Geometry check sheet. Reference: the model listing, model coordinates, mm. Round coordinates to 2 decimals unless told otherwise and drop trailing zeros. Order: outer loops, then holes, each group sorted by start corner. A loop starts at its lowest first (then second) coordinate and runs counter-clockwise, first axis right, second up. Notation, with made-up numbers: (-14.5, 46) - (9.5, 46) arc R21 ccw to (9.5, 73) - close; hole circle Ø9 at (56, 89). An arc over 180 degrees is marked (long way). Write each question's results on one line, items separated by ' | '.
```python
from build123d import *

# Parameters (mm, degrees)
SZKIC1_R                        = 3
DODANIE_WYCI_GNI_CIE1_DEPTH     = 65
DODANIE_WYCI_GNI_CIE2_START     = 65
SZKIC1_2_R                      = 3
DODANIE_WYCI_GNI_CIE2_DEPTH     = 120
SFAZOWANIE1_SIZE                = 1
SZKIC2_R                        = 1.05
WYTNIJ_WYCI_GNI_CIE1_DEPTH      = 4
WYTNIJ_WYCI_GNI_CIE1_DEPTH_BACK = 4


with BuildPart() as part:
    # Szkic1 → Dodanie-wyci_gni_cie1 (new body)
    with BuildSketch(Plane.XY):
        Circle(SZKIC1_R)
    extrude(amount=DODANIE_WYCI_GNI_CIE1_DEPTH)

    # Szkic1_2 → Dodanie-wyci_gni_cie2 (add)
    with BuildSketch(Plane.XY.offset(DODANIE_WYCI_GNI_CIE2_START)):
        Circle(SZKIC1_2_R)
    extrude(amount=-DODANIE_WYCI_GNI_CIE2_DEPTH)

    # Sfazowanie1
    sfazowanie1_edges = [part.edges().sort_by_distance(p)[0] for p in [
        (-3, 0, 65),
        (-3, 0, -55),
    ]]
    chamfer(sfazowanie1_edges, length=SFAZOWANIE1_SIZE)

    # Szkic2 → Wytnij-wyci_gni_cie1 (cut, two sides)
    with BuildSketch(Plane(origin=(0, 0, 0), x_dir=(1, 0, 0), z_dir=(0, 1, 0))) as wytnij_wyci_gni_cie1_sk:
        Circle(SZKIC2_R)
    extrude(amount=WYTNIJ_WYCI_GNI_CIE1_DEPTH, mode=Mode.SUBTRACT)
    extrude(wytnij_wyci_gni_cie1_sk.sketch, amount=-WYTNIJ_WYCI_GNI_CIE1_DEPTH_BACK, mode=Mode.SUBTRACT)


solid = part.part
```
(1) Section check B-B (z = 0). Record the cut outline in (x, y).
Answers follow:
outline: (-1.05, -2.81) - (-1.05, 2.81) arc R3 ccw to start; (1.05, -2.81) arc R3 ccw to (1.05, 2.81) - close
(2) Material ranges on line 1 (Z direction, x = 0, y = -1); line 2 (X direction, y = -2.25, z = 8.5); line 3 (X direction, y = -2.35, z = 0), recorded low to high.
Answers follow:
line 1: -55 to -1.05, 1.05 to 65 | line 2: -1.98 to 1.98 | line 3: -1.86 to -1.05, 1.05 to 1.86
(3) Section check C-C (z = 44). Record the cut outline in (x, y).
Answers follow:
outline: circle Ø6 at (0, 0)
(4) Section check A-A (x = 0). Record the cut outline in (y, z), then the cut area to 3 significant figures.
Answers follow:
outline: (-3, -54) - (-2, -55) - (2, -55) - (3, -54) - (3, -1.05) - (-3, -1.05) - close; (-3, 1.05) - (3, 1.05) - (3, 64) - (2, 65) - (-2, 65) - (-3, 64) - close | area: 705 mm²
(5) Depth check by flat-ended pin: pin 1 Ø2 at (y, z) = (2, -34) entering from -X; pin 2 Ø1.9 at (x, z) = (0, 0) entering from -Y; pin 3 Ø1.5 at (y, z) = (2, -22) entering from +X. Enter the tip coordinate at first touch or a pass-through.
Answers follow:
pin 1: x = -2.83 | pin 2: through | pin 3: x = 2.73
